Build history of the part. All positions in model axes, mm. A direction names the side the tool comes from. Round coordinates to 2 decimals unless told otherwise and drop trailing zeros. Loops run counter-clockwise (first coordinate to the right, second up) from the corner with the lowest first, then second, coordinate; pieces in that order, holes last. Notation, with made-up numbers: M 39.5,-31 L 63.5,-31 A28 ccw 63.5,-9 Z; hole C 14.5,-34 d2. An arc over 180 degrees is marked long. One line per item, written item: value.
```python
from build123d import *

# Parameters (mm, degrees)
ESQUISSE1_R             = 2.5
BASE_EXTRUSION_DEPTH    = 1.5
BASE_EXTRUSION_TAPER    = 8
CONG_1_R                = 0.75
CONG_2_R                = 0.25
ESQUISSE2_R             = 1.5
BOSS_EXTRU_1_DEPTH      = 10
CHANFREIN1_SIZE         = 0.5
ENL_V_MAT_EXTRU_1_DEPTH = 1
ESQUISSE5_W             = 0.5
ESQUISSE5_H             = 5.000243794
ENL_V_MAT_EXTRU_2_DEPTH = 0.75


with BuildPart() as part:
    # Esquisse1 → Base-Extrusion (new body)
    with BuildSketch(Plane.XY):
        Circle(ESQUISSE1_R)
    extrude(amount=BASE_EXTRUSION_DEPTH, taper=BASE_EXTRUSION_TAPER)

    # Congé1
    cong_1_edges = [part.edges().sort_by_distance(p)[0] for p in [
        (-2.289188748, 0, 1.5),
    ]]
    fillet(cong_1_edges, radius=CONG_1_R)

    # Congé2
    cong_2_edges = [part.edges().sort_by_distance(p)[0] for p in [
        (-2.5, 0, 0),
    ]]
    fillet(cong_2_edges, radius=CONG_2_R)

    # Esquisse2 → Boss.-Extru.1 (add)
    with BuildSketch(Plane(origin=(0, 0, 0), x_dir=(-1, 0, 0), z_dir=(0, 0, -1))):
        Circle(ESQUISSE2_R)
    extrude(amount=BOSS_EXTRU_1_DEPTH)

    # Chanfrein1
    chanfrein1_edges = [part.edges().sort_by_distance(p)[0] for p in [
        (1.5, 0, -10),
    ]]
    chamfer(chanfrein1_edges, length=CHANFREIN1_SIZE)

    # Esquisse4 → Enlèv. mat.-Extru.1 (cut)
    with BuildSketch(Plane.XY.offset(1.5)):
        with BuildLine():
            Line((-0.25, 1.75), (-0.25, 0.572821962))
            ThreePointArc((-0.25, 0.572821962), (-0.441941738, 0.441941738), (-0.572821962, 0.25))
            Line((-0.572821962, 0.25), (-1.75, 0.25))
            Line((-1.75, 0.25), (-1.75, -0.25))
            Line((-1.75, -0.25), (-0.572821962, -0.25))
            ThreePointArc((-0.572821962, -0.25), (-0.441941738, -0.441941738), (-0.25, -0.572821962))
            Line((-0.25, -0.572821962), (-0.25, -1.75))
            Line((-0.25, -1.75), (0.25, -1.75))
            Line((0.25, -1.75), (0.25, -0.572821962))
            ThreePointArc((0.25, -0.572821962), (0.441941738, -0.441941738), (0.572821962, -0.25))
            Line((0.572821962, -0.25), (1.75, -0.25))
            Line((1.75, -0.25), (1.75, 0.25))
            Line((1.75, 0.25), (0.572821962, 0.25))
            ThreePointArc((0.572821962, 0.25), (0.441941738, 0.441941738), (0.25, 0.572821962))
            Line((0.25, 0.572821962), (0.25, 1.75))
            Line((0.25, 1.75), (-0.25, 1.75))
        make_face()
    extrude(amount=-ENL_V_MAT_EXTRU_1_DEPTH, mode=Mode.SUBTRACT)

    # Esquisse5 → Enlèv. mat.-Extru.2 (cut)
    with BuildSketch(Plane.XY.offset(1.5)):
        with Locations((0, 0.01124212)):
            Rectangle(ESQUISSE5_W, ESQUISSE5_H)
    extrude(amount=-ENL_V_MAT_EXTRU_2_DEPTH, mode=Mode.SUBTRACT)


solid = part.part
```
Item 1: Drop flat-ended pins along their axis: P1, Ø0.8, axis at y = 1.5, z = 1, coming from the -X side; P2, Ø1.5, axis at y = 1, z = 0, coming from the -X side; P3, Ø1.5, axis at x = 2, z = -0.5, coming from the -Y side. Give the stop position or say it passes through.
Check values:
P1: stops at x = -2.1
P2: stops at x = -2.45
P3: stops at y = -1.85
Item 2: Which spindle directions (+Z, -Z, +X, -X, +Y, -Y) get a long thin tool onto all of the face, cutting with end or side? Do faces 5 (the face through (-0.25, -1, 1)), 6 (the face through (1, -1, 1.5)), 7 (the face through (-2, 0, 0)). Say none if no direction does.
Check values:
face 5: +Z
face 6: +Z, +X, -X, +Y, -Y
face 7: -Z
Item 3: Slice it at C-C, the plane z = -0.75. Give the cut face in (x, y).
Check values:
outline: C 0,0 d3
Item 4: Slice it at A-A, the plane x = 0. Give the cut face in (y, z).
Check values:
outline: M -2.46,0.28 A0.25 ccw -2.21,0 L -1.5,0 L -1.5,-9.5 L -1,-10 L 1,-10 L 1.5,-9.5 L 1.5,0 L 2.21,0 A0.25 ccw 2.46,0.28 L 2.39,0.75 L 1.75,0.75 L 1.75,0.5 L -1.75,0.5 L -1.75,0.75 L -2.39,0.75 Z
Item 5: Pull direction X, two halves, no side cores. Call faces 1 (the face through (1.5, 0.07, -4.68)), 2 (the face through (0.25, 1, 1)), 3 (the face through (0.25, -1, 1)), 4 (the face through (1, 1, 1.5)): pulls with the +X half, pulls with the -X half, needs draft (parallel to the pull), parting line crosses it, or undercut.
Check values:
face 1: parting line crosses it
face 2: undercut
face 3: undercut
face 4: needs draft
Item 6: Slice it at B-B, the plane y = 0. Give the cut face in (x, z), and give its area (3 significant figures).
Check values:
outline: M -2.46,0.28 A0.25 ccw -2.21,0 L -1.5,0 L -1.5,-9.5 L -1,-10 L 1,-10 L 1.5,-9.5 L 1.5,0 L 2.21,0 A0.25 ccw 2.46,0.28 L 2.38,0.85 A0.75 ccw 1.75,1.49 L 1.75,0.5 L -1.75,0.5 L -1.75,1.49 A0.75 ccw -2.38,0.85 Z
area: 33.2 mm2
Item 7: Wall check: line 1 along Z through (x, y) = (0.55, -1.5); line 2 along Z through (x, y) = (0.05, 0.2); line 3 along Y through (x, z) = (0.7, -0.5). Give the ranges that are in metal, low to high.
Check values:
line 1: z = 0 to 1.5
line 2: z = -10 to 0.5
line 3: y = -1.33 to 1.33
